Can you work these out from the model? Positions are in its coordinate system, mm. Face numbers are marked on the shaded views. A direction names the side the tool comes from. Give positions to 0.01 mm unless a question says otherwise; leave off trailing zeros. Loops run counter-clockwise (first coordinate to the right, second up) from the corner with the lowest first, then second, coordinate; pieces in that order, holes last. Notation, with made-up numbers: (-34.5, 36) - (-2.5, 36) arc R32 cw to (-2.5, 71) - close; hole circle Ø7 at (75.25, -33.5). An arc over 180 degrees is marked (long way). Write item = value, one per line.
from build123d import *

# Parameters (mm, degrees)
F2_SIZE  = 3.5
F3_R     = 5
F4_DEPTH = 19.001
F6_START = -5.3
F6_DEPTH = 8.3


with BuildPart() as f1:
    # F0 (on Front) → F1 (revolve)
    with BuildSketch(Plane.XZ):
        Polygon((0, 67.4), (0, 32.5), (5.2, 32.5), (5.2, 62), (23, 62), (23, 71.5), (39, 71.5), (39, 119.5), (19, 119.5), (19, 67.4), align=None)
    revolve(axis=Axis((17.3667171039, 0, 0), (1, 0, 0)))

    # F2
    f2_edges = [f1.edges().sort_by_distance(p)[0] for p in [
        (5.2, 0, -32.5),
    ]]
    chamfer(f2_edges, length=F2_SIZE)

    # F3 (on face) → F4 (cut, through all)
    with BuildSketch(Plane(origin=(19, 0, 0), x_dir=(0, -1, 0), z_dir=(-1, 0, 0))):
        with Locations((0, 50)):
            Circle(F3_R)
        with Locations((-50, 0)):
            Circle(F3_R)
        with Locations((50, 0)):
            Circle(F3_R)
        with Locations((0, -50)):
            Circle(F3_R)
    extrude(amount=F4_DEPTH, mode=Mode.SUBTRACT)

    # F5 (on face) → F6 (cut)
    with BuildSketch(Plane.YZ.offset(39).offset(F6_START)):
        Polygon((-46.1890190468, 38.2592231035), (-37.225138396, 38.2592231035), (-37.225138396, 47.0264043319), (-50.546871926, 49.8580262065), (-217.0100994408, 49.8580262065), (-217.0100994408, 38.2592231035), (-59.8083680284, 38.2592231035), (-46.7777463385, 41.0289672464), align=None)
        Polygon((-44.3662195739, 29.6836258198), (-46.1890190468, 38.2592231035), (-59.8083680284, 38.2592231035), (-222.6339746325, 3.6495720119), (-220.2224478679, -7.6957694146), (-66.4559514556, 24.9883083628), (-54.2859423014, 30.4067455387), (-53.1342179257, 27.8199302374), align=None)
        Polygon((-59.8083680284, 38.2592231035), (-46.1890190468, 38.2592231035), (-46.7777463385, 41.0289672464), align=None)
        Polygon((-50.546871926, 49.8580262065), (-37.225138396, 47.0264043319), (-37.225138396, 49.8580262065), align=None)
        Polygon((-37.225138396, 49.8580262065), (-37.225138396, 47.0264043319), (-28.4571400442, 45.1627087495), (-26.6343405713, 53.7383060332), (-39.0762349696, 59.2777943189), (-201.9018415736, 93.8874454105), (-204.3133683382, 82.5421039839), (-50.546871926, 49.8580262065), align=None)
        Polygon((-49.5682840636, 19.8107116499), (-53.1342179257, 27.8199302374), (-66.4559514556, 24.9883083628), (-218.5276768163, -42.7183859921), (-213.8100185785, -53.3144198809), (-70.1990909132, 10.6252846394), (-59.4215820929, 18.4556031433), (-57.757196515, 16.1647729251), align=None)
        Polygon((-66.4559514556, 24.9883083628), (-53.1342179257, 27.8199302374), (-54.2859423014, 30.4067455387), align=None)
        Polygon((-26.0456132796, 56.508050176), (-26.6343405713, 53.7383060332), (-18.44542812, 50.0923673084), (-14.8794942579, 58.1015858959), (-25.8977790364, 66.1068383731), (-177.9695043971, 133.8135327281), (-182.6871626349, 123.2174988393), (-39.0762349696, 59.2777943189), align=None)
        Polygon((-39.0762349696, 59.2777943189), (-26.6343405713, 53.7383060332), (-26.0456132796, 56.508050176), align=None)
        Polygon((-52.6039766848, 9.0719743186), (-57.757196515, 16.1647729251), (-70.1990909132, 10.6252846394), (-204.8706709112, -87.2193455428), (-198.053065503, -96.6029743675), (-70.8741932453, -4.2021150085), (-61.9602136106, 5.6978623307), (-59.8559084668, 3.8031374688), align=None)
        Polygon((-70.1990909132, 10.6252846394), (-57.757196515, 16.1647729251), (-59.4215820929, 18.4556031433), align=None)
        Polygon((-13.7277698822, 60.6884011972), (-14.8794942579, 58.1015858959), (-7.6275624759, 52.8327490461), (-2.4743426457, 59.9255476526), (-11.587465888, 70.0466963747), (-146.259045886, 167.8913265569), (-153.0766512942, 158.5076977322), (-25.8977790364, 66.1068383731), align=None)
        Polygon((-25.8977790364, 66.1068383731), (-14.8794942579, 58.1015858959), (-13.7277698822, 60.6884011972), align=None)
        Polygon((-53.3406231029, -2.0632518226), (-59.8559084668, 3.8031374688), (-70.8741932453, -4.2021150085), (-182.2598336087, -127.9084011684), (-173.640243101, -135.6695153217), (-68.4517532404, -18.8458620665), (-61.7908864754, -7.3089024071), (-59.3386299981, -8.7247133444), align=None)
        Polygon((-70.8741932453, -4.2021150085), (-59.8559084668, 3.8031374688), (-61.9602136106, 5.6978623307), align=None)
        Polygon((-0.8099570678, 62.2163778708), (-2.4743426457, 59.9255476526), (3.5236642494, 53.2640861308), (10.0389496133, 59.1304754222), (3.2292751225, 70.9251776233), (-108.156365241, 194.6314637832), (-116.7759557487, 186.8703496299), (-11.587465888, 70.0466963747), align=None)
        Polygon((-11.587465888, 70.0466963747), (-2.4743426457, 59.9255476526), (-0.8099570678, 62.2163778708), align=None)
        Polygon((-51.7460283347, -13.1083039586), (-59.3386299981, -8.7247133444), (-68.4517532404, -18.8458620665), (-151.6833669978, -163.0072458903), (-141.6385088571, -168.8066474418), (-63.0376431509, -32.6659545198), (-58.9210010956, -19.9962330377), (-56.2279686601, -20.8712523186), align=None)
        Polygon((-68.4517532404, -18.8458620665), (-59.3386299981, -8.7247133444), (-61.7908864754, -7.3089024071), align=None)
        Polygon((12.1432547571, 61.0252002841), (10.0389496133, 59.1304754222), (14.5208899387, 51.3675270621), (22.113491602, 55.7511176763), (17.9048813144, 68.703888273), (-65.326732443, 212.8652720968), (-75.3715905837, 207.0658705453), (3.2292751225, 70.9251776233), align=None)
        Polygon((3.2292751225, 70.9251776233), (10.0389496133, 59.1304754222), (12.1432547571, 61.0252002841), align=None)
        Polygon((-47.8898838233, -23.580460311), (-56.2279686601, -20.8712523186), (-63.0376431509, -32.6659545198), (-114.4776093915, -190.9818917712), (-103.4464921192, -194.5661190445), (-54.8684855676, -45.0583880119), (-53.4759852337, -31.809632332), (-50.65987528, -32.1056174151), align=None)
        Polygon((-63.0376431509, -32.6659545198), (-56.2279686601, -20.8712523186), (-58.9210010956, -19.9962330377), align=None)
        Polygon((24.5657480794, 57.1669286136), (22.113491602, 55.7511176763), (24.8834830587, 47.2259605721), (33.2215678954, 49.9351685644), (31.7979582757, 63.4799093273), (-19.6420079649, 221.7958465788), (-30.6731252372, 218.2116193056), (17.9048813144, 68.703888273), align=None)
        Polygon((17.9048813144, 68.703888273), (22.113491602, 55.7511176763), (24.5657480794, 57.1669286136), align=None)
        Polygon((-41.9407215877, -33.0220373961), (-50.65987528, -32.1056174151), (-54.8684855676, -45.0583880119), (-72.2686309303, -210.609712549), (-60.7333672843, -211.8221176131), (-44.3013118768, -55.4815537337), (-45.6938122107, -42.2327980539), (-42.877702257, -41.9368129708), align=None)
        Polygon((-54.8684855676, -45.0583880119), (-50.65987528, -32.1056174151), (-53.4759852337, -31.809632332), align=None)
        Polygon((35.914600331, 50.8101878453), (33.2215678954, 49.9351685644), (34.1585485648, 41.0203929898), (42.877702257, 41.9368129708), (44.3013118768, 55.4815537337), (26.9011665141, 221.0328782709), (15.3659028681, 219.8204732068), (31.7979582757, 63.4799093273), align=None)
        Polygon((31.7979582757, 63.4799093273), (33.2215678954, 49.9351685644), (35.914600331, 50.8101878453), align=None)
        Polygon((-34.1585485648, -41.0203929898), (-42.877702257, -41.9368129708), (-44.3013118768, -55.4815537337), (-26.9011665141, -221.0328782709), (-15.3659028681, -219.8204732068), (-31.7979582757, -63.4799093273), (-35.914600331, -50.8101878453), (-33.2215678954, -49.9351685644), align=None)
        Polygon((-44.3013118768, -55.4815537337), (-42.877702257, -41.9368129708), (-45.6938122107, -42.2327980539), align=None)
        Polygon((45.6938122107, 42.2327980539), (42.877702257, 41.9368129708), (41.9407215877, 33.0220373961), (50.65987528, 32.1056174151), (54.8684855676, 45.0583880119), (72.2686309303, 210.609712549), (60.7333672843, 211.8221176131), (44.3013118768, 55.4815537337), align=None)
        Polygon((44.3013118768, 55.4815537337), (42.877702257, 41.9368129708), (45.6938122107, 42.2327980539), align=None)
        Polygon((-24.8834830587, -47.2259605721), (-33.2215678954, -49.9351685644), (-31.7979582757, -63.4799093273), (19.6420079649, -221.7958465788), (30.6731252372, -218.2116193056), (-17.9048813144, -68.703888273), (-24.5657480794, -57.1669286136), (-22.113491602, -55.7511176763), align=None)
        Polygon((-31.7979582757, -63.4799093273), (-33.2215678954, -49.9351685644), (-35.914600331, -50.8101878453), align=None)
        Polygon((53.4759852337, 31.809632332), (50.65987528, 32.1056174151), (47.8898838233, 23.580460311), (56.2279686601, 20.8712523186), (63.0376431509, 32.6659545198), (114.4776093915, 190.9818917712), (103.4464921192, 194.5661190445), (54.8684855676, 45.0583880119), align=None)
        Polygon((54.8684855676, 45.0583880119), (50.65987528, 32.1056174151), (53.4759852337, 31.809632332), align=None)
        Polygon((-14.5208899387, -51.3675270621), (-22.113491602, -55.7511176763), (-17.9048813144, -68.703888273), (65.326732443, -212.8652720968), (75.3715905837, -207.0658705453), (-3.2292751225, -70.9251776233), (-12.1432547571, -61.0252002841), (-10.0389496133, -59.1304754222), align=None)
        Polygon((-17.9048813144, -68.703888273), (-22.113491602, -55.7511176763), (-24.5657480794, -57.1669286136), align=None)
        Polygon((58.9210010956, 19.9962330377), (56.2279686601, 20.8712523186), (51.7460283347, 13.1083039586), (59.3386299981, 8.7247133444), (68.4517532404, 18.8458620665), (151.6833669978, 163.0072458903), (141.6385088571, 168.8066474418), (63.0376431509, 32.6659545198), align=None)
        Polygon((63.0376431509, 32.6659545198), (56.2279686601, 20.8712523186), (58.9210010956, 19.9962330377), align=None)
        Polygon((-3.5236642494, -53.2640861308), (-10.0389496133, -59.1304754222), (-3.2292751225, -70.9251776233), (108.156365241, -194.6314637832), (116.7759557487, -186.8703496299), (11.587465888, -70.0466963747), (0.8099570678, -62.2163778708), (2.4743426457, -59.9255476526), align=None)
        Polygon((-3.2292751225, -70.9251776233), (-10.0389496133, -59.1304754222), (-12.1432547571, -61.0252002841), align=None)
        Polygon((61.7908864754, 7.3089024071), (59.3386299981, 8.7247133444), (53.3406231029, 2.0632518226), (59.8559084668, -3.8031374688), (70.8741932453, 4.2021150085), (182.2598336087, 127.9084011684), (173.640243101, 135.6695153217), (68.4517532404, 18.8458620665), align=None)
        Polygon((68.4517532404, 18.8458620665), (59.3386299981, 8.7247133444), (61.7908864754, 7.3089024071), align=None)
        Polygon((7.6275624759, -52.8327490461), (2.4743426457, -59.9255476526), (11.587465888, -70.0466963747), (146.259045886, -167.8913265569), (153.0766512942, -158.5076977322), (25.8977790364, -66.1068383731), (13.7277698822, -60.6884011972), (14.8794942579, -58.1015858959), align=None)
        Polygon((11.587465888, -70.0466963747), (2.4743426457, -59.9255476526), (0.8099570678, -62.2163778708), align=None)
        Polygon((61.9602136106, -5.6978623307), (59.8559084668, -3.8031374688), (52.6039766848, -9.0719743186), (57.757196515, -16.1647729251), (70.1990909132, -10.6252846394), (204.8706709112, 87.2193455428), (198.053065503, 96.6029743675), (70.8741932453, 4.2021150085), align=None)
        Polygon((70.8741932453, 4.2021150085), (59.8559084668, -3.8031374688), (61.9602136106, -5.6978623307), align=None)
        Polygon((18.44542812, -50.0923673084), (14.8794942579, -58.1015858959), (25.8977790364, -66.1068383731), (177.9695043971, -133.8135327281), (182.6871626349, -123.2174988393), (39.0762349696, -59.2777943189), (26.0456132796, -56.508050176), (26.6343405713, -53.7383060332), align=None)
        Polygon((25.8977790364, -66.1068383731), (14.8794942579, -58.1015858959), (13.7277698822, -60.6884011972), align=None)
        Polygon((59.4215820929, -18.4556031433), (57.757196515, -16.1647729251), (49.5682840636, -19.8107116499), (53.1342179257, -27.8199302374), (66.4559514556, -24.9883083628), (218.5276768163, 42.7183859921), (213.8100185785, 53.3144198809), (70.1990909132, -10.6252846394), align=None)
        Polygon((70.1990909132, -10.6252846394), (57.757196515, -16.1647729251), (59.4215820929, -18.4556031433), align=None)
        Polygon((28.4571400442, -45.1627087495), (26.6343405713, -53.7383060332), (39.0762349696, -59.2777943189), (201.9018415736, -93.8874454105), (204.3133683382, -82.5421039839), (50.546871926, -49.8580262065), (37.225138396, -49.8580262065), (37.225138396, -47.0264043319), align=None)
        Polygon((39.0762349696, -59.2777943189), (26.6343405713, -53.7383060332), (26.0456132796, -56.508050176), align=None)
        Polygon((54.2859423014, -30.4067455387), (53.1342179257, -27.8199302374), (44.3662195739, -29.6836258198), (46.1890190468, -38.2592231035), (59.8083680284, -38.2592231035), (222.6339746325, -3.6495720119), (220.2224478679, 7.6957694146), (66.4559514556, -24.9883083628), align=None)
        Polygon((66.4559514556, -24.9883083628), (53.1342179257, -27.8199302374), (54.2859423014, -30.4067455387), align=None)
        Polygon((37.225138396, -38.2592231035), (37.225138396, -47.0264043319), (50.546871926, -49.8580262065), (217.0100994408, -49.8580262065), (217.0100994408, -38.2592231035), (59.8083680284, -38.2592231035), (46.7777463385, -41.0289672464), (46.1890190468, -38.2592231035), align=None)
        Polygon((50.546871926, -49.8580262065), (37.225138396, -47.0264043319), (37.225138396, -49.8580262065), align=None)
        Polygon((59.8083680284, -38.2592231035), (46.1890190468, -38.2592231035), (46.7777463385, -41.0289672464), align=None)
    extrude(amount=-F6_DEPTH, mode=Mode.SUBTRACT)


solid = f1.part
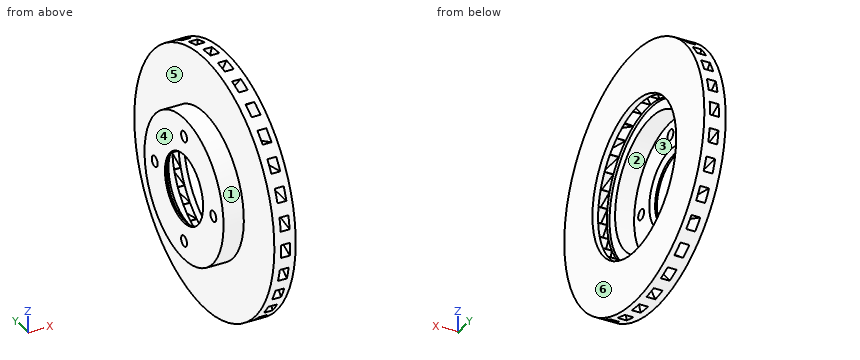
Q1. We'd pull the mould along Y, two halves only. Please class the marked faces 1, 2, 3 and 4: released by +Y, released by -Y, zero draft, split by the parting line, or undercut.
Output:
face_1 = split by the parting line
face_2 = undercut
face_3 = undercut
face_4 = zero draft
Q2. Imagine slicing it at A-A, the plane x = 9. Write out the boundary of the cut face in (y, z), then the cut area to 3 significant figures.
Output:
outline = circle Ø134.8 at (0, 0); hole circle Ø124 at (0, 0)
area = 2,200 mm2
Q3. Which directions (+Z, -Z, +X, -X, +Y, -Y) give clear straight access to the entire face, cutting with the end or side of a thin tool? Please do the marked faces 5 and 6.
Output:
face_5 = -X
face_6 = +Z, -Z, +X, +Y, -Y
Q4. For pin 1 (4 mm diameter, centred on y = 52, z = 55, fed in from -X); pin 2 (2 mm diameter, centred on x = 34, z = -27.5, fed in from +Y); pin 3 (2 mm diameter, centred on x = 21, y = 78, fed in from -Z), each with a flat end and sliding along its axis, tell me the tip position at first contact or that it passes through.
Output:
pin_1 = 19
pin_2 = 116.52
pin_3 = -91.39
Q5. I need wall thicknesses on L1, parallel to X at y = 19, z = -79; L2, parallel to Y at x = 35.75, z = 0; L3, parallel to Z at x = 37.5, y = -3.5. Which ranges of each line are inside material? Lowest first, please.
Output:
L1 = 19 to 25.4, 33.7 to 39
L2 = -119.5 to -71.5, 71.5 to 119.5
L3 = -119.45 to -71.41, 71.41 to 119.45
